Build history of the part. All positions in model axes, mm. Face numbers are marked on the shaded views. A direction names the side the tool comes from. Coordinates: 2 decimals unless noted, no trailing zeros. Loops run counter-clockwise (first coordinate to the right, second up) from the corner with the lowest first, then second, coordinate; pieces in that order, holes last.
(1) Flat gauge pins, fed straight in: P1, Ø10, axis at x = 95, y = 33.5, coming from the +Z side; P2, Ø9, axis at y = 4.5, z = 82, coming from the -X side; P3, Ø4, axis at x = 142.5, z = 51.5, coming from the +Y side; P4, Ø3, axis at x = 83, z = 19.5, coming from the +Y side. Where does each tip first touch, or does it go through?
(2) Slice it at C-C (z = 99). Give the cut face in (x, y).
(3) Slice it at D-D (x = 49). Give the cut face in (y, z).
(4) Slice it at A-A (y = 22.5). Give the cut face in (x, z) (3 decimals).
(5) Wall check: L1, parallel to Y at x = 149.5, z = 45; L2, parallel to Y at x = 45, z = 50; L3, parallel to Y at x = 64, z = 30.5. Give the ranges that are in metal, low to high.
(6) Slice it at B-B (y = 12.5). Give the cut face in (x, z), and give its area (3 significant figures).
(7) Tool access for the marked faces 1 and 2: list every direction of +Z, -Z, +X, -X, +Y, -Y with a clear straight run to the whole face (end or side of a thin tool).
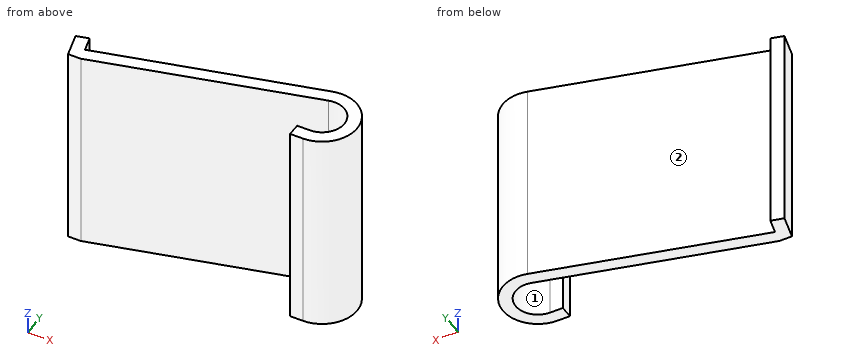
from build123d import *

# Parameters (mm, degrees)
PAD_DEPTH = 130


with BuildPart() as part:
    # Sketch → Pad (new body)
    with BuildSketch(Plane.XY):
        with BuildLine():
            Line((0, 0), (8, 0))
            Line((8, 0), (143.800384, 35.063508))
            ThreePointArc((147.237874, 8), (160.878343, 23.482615), (143.800384, 35.063508))
            Line((139.237875, 8), (147.237874, 8))
            Line((139.237875, 8), (139.237875, 0))
            Line((139.237875, 0), (147.237875, 0))
            ThreePointArc((147.237875, 0), (168.81458, 24.49065), (141.800384, 42.809475))
            Line((6.245967, 7.809475), (141.800384, 42.809475))
            Line((3.745967, 17.491933), (6.245967, 7.809475))
            Line((-4, 15.491933), (3.745967, 17.491933))
            Line((0, 0), (-4, 15.491933))
        make_face()
    extrude(amount=PAD_DEPTH)


solid = part.part
Response values:
1. P1: stops at z = 130
1. P2: stops at x = -2.32
1. P3: stops at y = 43.33
1. P4: stops at y = 28.01
2. outline: (-4, 15.49) - (0, 0) - (8, 0) - (143.8, 35.06) arc R13.75 cw (long way) to (147.24, 8) - (139.24, 8) - (139.24, 0) - (147.24, 0) arc R21.75 ccw (long way) to (141.8, 42.81) - (6.25, 7.81) - (3.75, 17.49) - close
3. outline: (10.59, 0) - (18.85, 0) - (18.85, 130) - (10.59, 130) - close
4. outline: (63.142, 0) - (95.142, 0) - (95.142, 130) - (63.142, 130) - close; (160.967, 0) - (168.975, 0) - (168.975, 130) - (160.967, 130) - close
5. L1: y = 0.12 to 8.19, 35.31 to 43.38
5. L2: y = 9.55 to 17.82
5. L3: y = 14.46 to 22.72
6. outline: (-3.23, 0) - (5.03, 0) - (5.03, 130) - (-3.23, 130) - close; (24.41, 0) - (56.41, 0) - (56.41, 130) - (24.41, 130) - close; (157.41, 0) - (166.92, 0) - (166.92, 130) - (157.41, 130) - close
6. area: 6,470 mm2
7. face 1: +Z, -Z
7. face 2: +Z, -Z, +Y
